Work out the finished part from the listing and answer in its coordinate system (mm). A direction names the side the tool comes from. Round coordinates to 2 decimals unless told otherwise and drop trailing zeros. Write each loop counter-clockwise with the first axis right and the second up, starting at its lowest first coordinate (ties: lowest second). Pieces come first, ordered by that corner, then holes. Notation, with made-up numbers: (46.25, 15) -> (96.25, 15) arc R23 ccw to (96.25, 47) -> close; hole circle Ø8 at (67.25, 80). An arc over 180 degrees is marked (long way). One line per item, written item: value.
```python
from build123d import *

# Parameters (mm, degrees)
BASPROSKE_W             = 10
BASPROSKE_H             = 19
TOOTHCUT_DEPTH          = 29.670542374
TEETHCUTS_COUNT         = 17
TEETHCUTS_ANGLE         = 338.823529412
BORSKE_R                = 2.5
BORE_DEPTH              = 50.0018796
SKETCH1_W               = 10
SKETCH1_H               = 40
CUT_EXTRUDE1_DEPTH      = 20
CUT_EXTRUDE1_DEPTH_BACK = 20
BOSS_EXTRUDE1_DEPTH     = 5
SKETCH5_R               = 4.75
SKETCH5_R_2             = 2.5
CUT_EXTRUDE2_DEPTH      = 3
SKETCH6_R               = 1.5
CUT_EXTRUDE3_DEPTH      = 68.251600881
SKETCH7_R               = 1.5
CUT_EXTRUDE4_DEPTH      = 3
FILLET1_R               = 4.5
FILLET2_R               = 4.5


with BuildPart() as part:
    # BasProSke → Base-Revolve (revolve)
    with BuildSketch(Plane(origin=(0, 0, 0), x_dir=(1, 0, 0), z_dir=(0, 1, 0)), mode=Mode.PRIVATE) as base_revolve_sk:
        with Locations((5, 9.5)):
            Rectangle(BASPROSKE_W, BASPROSKE_H)
    revolve(base_revolve_sk.sketch.rotate(Axis((-10, 0, 0), (1, 0, 0)), 180), axis=Axis((-10, 0, 0), (1, 0, 0)))

    # TooCutSke → ToothCut (cut, through all)
    with BuildSketch(Plane(origin=(0, 0, 0), x_dir=(0, 0, -1), z_dir=(1, 0, 0))):
        with BuildLine():
            ThreePointArc((1.020352389, 14.463052306), (0, 14.499), (-1.020352389, 14.463052306))
            ThreePointArc((-1.020352389, 14.463052306), (-1.632621885, 16.804485203), (-3.026143023, 18.783192049))
            ThreePointArc((-3.026143023, 18.783192049), (0, 19.0254), (3.026143023, 18.783192049))
            ThreePointArc((3.026143023, 18.783192049), (1.632621885, 16.804485203), (1.020352389, 14.463052306))
        make_face()
    toothcut = extrude(amount=TOOTHCUT_DEPTH, mode=Mode.SUBTRACT)

    # TeethCuts: ToothCut ×17 about axis
    teethcuts_axis = Axis((-10, 0, 0), (1, 0, 0))
    for i in range(1, TEETHCUTS_COUNT):
        add(toothcut.rotate(teethcuts_axis, i * TEETHCUTS_ANGLE / (TEETHCUTS_COUNT - 1)), mode=Mode.SUBTRACT)

    # BorSke → Bore (cut, symmetric)
    with BuildSketch(Plane(origin=(0, 0, 0), x_dir=(0, 0, -1), z_dir=(1, 0, 0))):
        with Locations(Location((0, 0, 0), (0, 0, 180))):
            Circle(BORSKE_R)
    extrude(amount=BORE_DEPTH, both=True, mode=Mode.SUBTRACT)

    # Sketch1 → Cut-Extrude1 (cut, two sides)
    with BuildSketch(Plane.XY) as cut_extrude1_sk:
        Rectangle(SKETCH1_W, SKETCH1_H)
    extrude(amount=CUT_EXTRUDE1_DEPTH, mode=Mode.SUBTRACT)
    extrude(cut_extrude1_sk.sketch, amount=-CUT_EXTRUDE1_DEPTH_BACK, mode=Mode.SUBTRACT)

    # Sketch4 → Boss-Extrude1 (add)
    with BuildSketch(Plane(origin=(10, 0, 0), x_dir=(0, 0, -1), z_dir=(1, 0, 0))):
        with BuildLine():
            Line((5, 0), (5, 47.113248654))
            Line((5, 47.113248654), (14.820508076, 52.783121635))
            Line((14.820508076, 52.783121635), (14.820508076, 64.330127019))
            Line((14.820508076, 64.330127019), (-5, 52.886751346))
            Line((-5, 52.886751346), (-5, 0))
            Line((-5, 0), (-2.5, 0))
            ThreePointArc((-2.5, 0), (0, 2.5), (2.5, 0))
            Line((2.5, 0), (5, 0))
        make_face()
    extrude(amount=-BOSS_EXTRUDE1_DEPTH)

    # Sketch5 → Cut-Extrude2 (cut)
    with BuildSketch(Plane.ZY.offset(-5)):
        with Locations(Location((0, 0, 0), (0, 0, 270))):
            Circle(SKETCH5_R)
        Circle(SKETCH5_R_2, mode=Mode.SUBTRACT)
    extrude(amount=-CUT_EXTRUDE2_DEPTH, mode=Mode.SUBTRACT)

    # Sketch6 → Cut-Extrude3 (cut, through all)
    with BuildSketch(Plane.ZY.offset(-5)):
        with Locations(Location((-11.320508076, 57.330127019, 0), (0, 0, 270))):
            Circle(SKETCH6_R)
    extrude(amount=-CUT_EXTRUDE3_DEPTH, mode=Mode.SUBTRACT)

    # Sketch7 → Cut-Extrude4 (cut)
    with BuildSketch(Plane.ZY.offset(-5)):
        with BuildLine():
            Line((-5.551409088, 58.978610224), (-14.820508076, 64.330127019))
            Line((-14.820508076, 64.330127019), (-14.820508076, 52.783121635))
            Line((-14.820508076, 52.783121635), (-12.5101794, 51.449252752))
            ThreePointArc((-12.5101794, 51.449252752), (-6.914194944, 53.257731583), (-5.551409088, 58.978610224))
        make_face()
        with Locations(Location((-11.320508076, 57.330127019, 0), (0, 0, 270))):
            Circle(SKETCH7_R, mode=Mode.SUBTRACT)
    extrude(amount=-CUT_EXTRUDE4_DEPTH, mode=Mode.SUBTRACT)

    # Fillet1
    fillet1_edges = [part.edges().sort_by_distance(p)[0] for p in [
        (9, 52.783121635, -14.820508076),
        (9, 64.330127019, -14.820508076),
    ]]
    fillet(fillet1_edges, radius=FILLET1_R)

    # Fillet2
    fillet2_edges = [part.edges().sort_by_distance(p)[0] for p in [
        (6.5, 51.449252752, -12.5101794),
    ]]
    fillet(fillet2_edges, radius=FILLET2_R)


solid = part.part
```
(1) Find section A-A on y = 32.5. Give the vertices of the cut face in (x, z).
Reported:
outline: (5, -5) -> (10, -5) -> (10, 5) -> (5, 5) -> close
(2) Flat-ended cylindrical pins translate along their axes: pin 1 Ø1.5 at (x, y) = (8, -8) entering from -Z; pin 2 Ø3 at (y, z) = (1.5, 1) entering from -X; pin 3 Ø1.5 at (x, y) = (7, 25) entering from -Z. Find the tip coordinate at first contact, or state that the pin passes through.
Reported:
pin 1: stops at z = -17.22
pin 2: stops at x = 8
pin 3: stops at z = -5
(3) A tool of negligible diameter and unlimited length cuts with its end or side. For faces 5 (the face through (7.465, 15.092, -7.606)), 6 (the face through (8.646, 49.268, -8.732)), 7 (the face through (6.48, 3.77, -2.89)), 8 (the face through (7.46, -6.14, 15.68)), from which of +Z, -Z, +X, -X, +Y, -Y can it reach the whole face along a straight path? Write none if from no direction.
Reported:
face 5: +X, -X
face 6: -Z, +X, -X
face 7: -X
face 8: +Z, +X, -X
(4) Consider probe 1 along Y at (x, z) = (8.3, 15); probe 2 along Y at (x, z) = (9.3, 16); probe 3 along Z at (x, y) = (7.55, 50.5). Determine where each line is inside the solid, lowest interval first.
Reported:
probe 1: y = -8.93 to -5.63, -3.09 to 0.31, 2.51 to 5.96, 9.99 to 11.66
probe 2: y = -8.97 to -6.43, -3.1 to 0.17, 2.87 to 6.03
probe 3: z = -7.34 to 5
(5) For a pull along Z with two mould halves and no side action, classify faces 1 (the face through (10, 20, 0)), 2 (the face through (7.46, -6.18, -15.73)), 3 (the face through (7.465, -8.828, 14.412)), 4 (the face through (7.465, 3.185, 16.598)) as pulls with the +Z half, pulls with the -Z half, needs draft (parallel to the pull), parting line crosses it, or undercut.
Reported:
face 1: needs draft
face 2: pulls with the -Z half
face 3: undercut
face 4: pulls with the +Z half
(6) Find section B-B on x = 9.1. Give the number of separate pieces and of enclosed holes in the cut face, plus the area to 3 significant figures.
Reported:
separate pieces: 1
enclosed holes: 2
area: 1,330 mm2
(7) Find section C-C on y = -11. Give the vertices of the cut face in (x, z).
Reported:
outline: (5, -12.18) -> (10, -12.18) -> (10, 12.18) -> (5, 12.18) -> close
